```python
from build123d import *

# Parameters (mm, degrees)
SKETCH1_W                      = 260
SKETCH1_H                      = 49
BOSS_EXTRUDE1_DEPTH            = 6
SKETCH2_W                      = 117
SKETCH2_H                      = 6
CUT_EXTRUDE1_DEPTH             = 140.057542046
SKETCH5_W                      = 3.4
SKETCH5_H                      = 6
CUT_EXTRUDE2_REACH             = 141.058
SKETCH6_W                      = 6
SKETCH6_H                      = 23
SKETCH7_W                      = 80
SKETCH7_H                      = 6
BOSS_EXTRUDE2_DEPTH            = 6
SKETCH8_R                      = 20
SKETCH8_R_2                    = 8.5
CUT_EXTRUDE3_DEPTH             = 6
SKETCH9_R                      = 5.75
BOSS_EXTRUDE3_DEPTH            = 6
CIRPATTERN1_COUNT              = 5
SKETCH11_W                     = 1.4351
SKETCH11_H                     = 6
F_6_40_TAPPED_HOLE1_AT_2_COUNT = 2
F_6_40_TAPPED_HOLE1_AT_2_PITCH = 32
F_6_40_TAPPED_HOLE1_AT_3_COUNT = 2
F_6_40_TAPPED_HOLE1_AT_3_PITCH = 45.254833996
F_6_40_TAPPED_HOLE1_AT_4_COUNT = 2
F_6_40_TAPPED_HOLE1_AT_4_PITCH = 32
SKETCH12_R                     = 1.4351
SKETCH12_R_2                   = 3.4
SKETCH12_R_3                   = 5.75
CUT_EXTRUDE4_DEPTH             = 6


with BuildPart() as part:
    # Sketch1 → Boss-Extrude1 (new body)
    with BuildSketch(Plane.XY):
        with Locations((0, 24.5)):
            Rectangle(SKETCH1_W, SKETCH1_H)
    extrude(amount=BOSS_EXTRUDE1_DEPTH)

    # Sketch2 → Cut-Extrude1 (cut, through all)
    with BuildSketch(Plane(origin=(0, 0, 0), x_dir=(-1, 0, 0), z_dir=(0, 0, -1))):
        with Locations((-71.5, 46)):
            Rectangle(SKETCH2_W, SKETCH2_H)
        with Locations((71.5, 46)):
            Rectangle(SKETCH2_W, SKETCH2_H)
    extrude(amount=-CUT_EXTRUDE1_DEPTH, mode=Mode.SUBTRACT)

    # Sketch5 → M8x1.25 Tapped Hole1 (revolve, cut)
    with BuildSketch(Plane(origin=(0, 39, 0), x_dir=(0, 1, 0), z_dir=(1, 0, 0))):
        with Locations((1.7, 3)):
            Rectangle(SKETCH5_W, SKETCH5_H)
    revolve(axis=Axis((0, 39, -6.35), (0, 0, 1)), mode=Mode.SUBTRACT)

    # Sketch6 → Cut-Extrude2 (cut, up to next)
    with BuildSketch(Plane(origin=(0, 0, 0), x_dir=(-1, 0, 0), z_dir=(0, 0, -1)), mode=Mode.PRIVATE) as cut_extrude2_sk1:
        with Locations((-127, 31.5)):
            Rectangle(SKETCH6_W, SKETCH6_H)
    cut_extrude2_tool1 = extrude(cut_extrude2_sk1.sketch, amount=-CUT_EXTRUDE2_REACH, mode=Mode.PRIVATE) & part.part
    # Sketch6 → Cut-Extrude2 (cut, up to next)
    with BuildSketch(Plane(origin=(0, 0, 0), x_dir=(-1, 0, 0), z_dir=(0, 0, -1)), mode=Mode.PRIVATE) as cut_extrude2_sk2:
        with Locations((127, 31.5)):
            Rectangle(SKETCH6_W, SKETCH6_H)
    cut_extrude2_tool2 = extrude(cut_extrude2_sk2.sketch, amount=-CUT_EXTRUDE2_REACH, mode=Mode.PRIVATE) & part.part
    add(cut_extrude2_tool1.solids().sort_by_distance((127, 31.5, 0))[0], mode=Mode.SUBTRACT)
    add(cut_extrude2_tool2.solids().sort_by_distance((-127, 31.5, 0))[0], mode=Mode.SUBTRACT)

    # Sketch7 → Boss-Extrude2 (add)
    with BuildSketch(Plane(origin=(0, 0, 0), x_dir=(-1, 0, 0), z_dir=(0, 0, -1))):
        with Locations((0, -3)):
            Rectangle(SKETCH7_W, SKETCH7_H)
    extrude(amount=-BOSS_EXTRUDE2_DEPTH)

    # Sketch8 → Cut-Extrude3 (cut)
    with BuildSketch(Plane(origin=(0, 0, 0), x_dir=(-1, 0, 0), z_dir=(0, 0, -1))):
        with Locations((-85, 21.5)):
            Circle(SKETCH8_R)
        with Locations((-85, 21.5)):
            Circle(SKETCH8_R_2, mode=Mode.SUBTRACT)
    extrude(amount=-CUT_EXTRUDE3_DEPTH, mode=Mode.SUBTRACT)


with BuildPart() as cut_extrude3_piece_1:
    # of the separate pieces the step leaves, piece 1, a body of its own (cut_extrude3_pieces)
    add(part.part.solids().sort_by_distance((130, 0, 0))[0])



with BuildPart() as cut_extrude3_piece_2:
    # of the separate pieces the step leaves, piece 2, a body of its own (cut_extrude3_pieces)
    add(part.part.solids().sort_by_distance((76.5, 21.5, 0))[0])


with BuildPart() as cut_extrude3_piece_1_1:
    add(cut_extrude3_piece_1.part)

    add(cut_extrude3_piece_2.part)  # Boss-Extrude3 merges Cut-Extrude3 piece 2
    # Sketch9 → Boss-Extrude3 (add)
    with BuildSketch(Plane(origin=(0, 0, 0), x_dir=(-1, 0, 0), z_dir=(0, 0, -1))):
        with BuildLine():
            ThreePointArc((-100.761482737, 35.377163324), (-88.82060414, 26.758610463), (-93.327400585, 40.778340164))
            ThreePointArc((-93.327400585, 40.778340164), (-97.343490298, 38.489356882), (-100.761482737, 35.377163324))
        make_face()
        with Locations((-93.375939845, 33.02849217)):
            Circle(SKETCH9_R, mode=Mode.SUBTRACT)
    boss_extrude3 = extrude(amount=-BOSS_EXTRUDE3_DEPTH)

    # CirPattern1: Boss-Extrude3 ×5 about axis
    cirpattern1_axis = Axis((85, 21.5, 0), (0, 0, -1))
    for i in range(1, CIRPATTERN1_COUNT):
        add(boss_extrude3.rotate(cirpattern1_axis, i * 360 / CIRPATTERN1_COUNT))

    # Sketch11 → #6-40 Tapped Hole1 (revolve, cut)
    with BuildSketch(Plane(origin=(101, 37.5, 0), x_dir=(0, 1, 0), z_dir=(1, 0, 0))):
        with Locations((0.71755, 3)):
            Rectangle(SKETCH11_W, SKETCH11_H)
    f_6_40_tapped_hole1 = revolve(axis=Axis((101, 37.5, -6.35), (0, 0, 1)), mode=Mode.SUBTRACT)

    # #6-40 Tapped Hole1 at 2: #6-40 Tapped Hole1 ×2
    with Locations(*[(-i * F_6_40_TAPPED_HOLE1_AT_2_PITCH, 0, 0) for i in range(1, F_6_40_TAPPED_HOLE1_AT_2_COUNT)]):
        add(f_6_40_tapped_hole1, mode=Mode.SUBTRACT)

    # #6-40 Tapped Hole1 at 3: #6-40 Tapped Hole1 ×2
    with Locations(*[Vector(-0.7071067811865476, -0.7071067811865476, 0) * (i * F_6_40_TAPPED_HOLE1_AT_3_PITCH) for i in range(1, F_6_40_TAPPED_HOLE1_AT_3_COUNT)]):
        add(f_6_40_tapped_hole1, mode=Mode.SUBTRACT)

    # #6-40 Tapped Hole1 at 4: #6-40 Tapped Hole1 ×2
    with Locations(*[(0, -i * F_6_40_TAPPED_HOLE1_AT_4_PITCH, 0) for i in range(1, F_6_40_TAPPED_HOLE1_AT_4_COUNT)]):
        add(f_6_40_tapped_hole1, mode=Mode.SUBTRACT)

    # Sketch12 → Cut-Extrude4 (cut)
    with BuildSketch(Plane(origin=(0, 0, 0), x_dir=(-1, 0, 0), z_dir=(0, 0, -1))):
        with Locations(Location((101, 37.5, 0), (0, 0, 180))):
            Circle(SKETCH12_R)
        with Locations((0, 39)):
            Circle(SKETCH12_R_2)
        with Locations((-93.375939845, 33.02849217)):
            Circle(SKETCH12_R_3)
        with Locations(Location((-76.624060155, 33.02849217, 0), (0, 0, 288))):
            Circle(SKETCH12_R_3)
        with Locations(Location((-71.447444643, 17.09650783, 0), (0, 0, 216))):
            Circle(SKETCH12_R_3)
        with Locations(Location((-85, 7.25, 0), (0, 0, 144))):
            Circle(SKETCH12_R_3)
        with Locations(Location((-98.552555357, 17.09650783, 0), (0, 0, 72))):
            Circle(SKETCH12_R_3)
        with Locations((-101, 5.5)):
            Circle(SKETCH12_R)
        with Locations((-69, 5.5)):
            Circle(SKETCH12_R)
        with Locations((-69, 37.5)):
            Circle(SKETCH12_R)
        with Locations((-101, 37.5)):
            Circle(SKETCH12_R)
        with Locations(Location((69, 37.5, 0), (0, 0, 180))):
            Circle(SKETCH12_R)
        with Locations(Location((69, 5.5, 0), (0, 0, 180))):
            Circle(SKETCH12_R)
        with Locations(Location((101, 5.5, 0), (0, 0, 180))):
            Circle(SKETCH12_R)
        with Locations(Location((98.552555357, 17.09650783, 0), (0, 0, 180))):
            Circle(SKETCH12_R_3)
        with Locations(Location((85, 7.25, 0), (0, 0, 180))):
            Circle(SKETCH12_R_3)
        with Locations(Location((71.447444643, 17.09650783, 0), (0, 0, 180))):
            Circle(SKETCH12_R_3)
        with Locations(Location((76.624060155, 33.02849217, 0), (0, 0, 180))):
            Circle(SKETCH12_R_3)
        with Locations(Location((93.375939845, 33.02849217, 0), (0, 0, 180))):
            Circle(SKETCH12_R_3)
        with BuildLine():
            ThreePointArc((-78.722018184, 40.489127003), (-83.633443041, 36.334706252), (-83.715608088, 29.902400694))
            ThreePointArc((-83.715608088, 29.902400694), (-85, 30), (-86.284391912, 29.902400694))
            ThreePointArc((-86.284391912, 29.902400694), (-86.366556959, 36.334706252), (-91.277981816, 40.489127003))
            ThreePointArc((-91.277981816, 40.489127003), (-85, 41.5), (-78.722018184, 40.489127003))
        make_face()
        with BuildLine():
            ThreePointArc((-65.000263954, 21.397247437), (-65.978869674, 27.680339887), (-68.880270097, 33.338678467))
            ThreePointArc((-68.880270097, 33.338678467), (-71.313645276, 27.383849239), (-77.405740996, 25.318013906))
            ThreePointArc((-77.405740996, 25.318013906), (-76.916019611, 24.126644452), (-76.611943139, 22.87495531))
            ThreePointArc((-76.611943139, 22.87495531), (-70.469066627, 24.784503438), (-65.000263954, 21.397247437))
        make_face()
        with BuildLine():
            ThreePointArc((-78.917465173, 2.447368421), (-73.244294954, 5.319660113), (-68.759477215, 9.827578672))
            ThreePointArc((-68.759477215, 9.827578672), (-75.174810639, 10.301712562), (-79.022097904, 15.45726167))
            ThreePointArc((-79.022097904, 15.45726167), (-80.003825356, 14.623355548), (-81.100287673, 13.947368421))
            ThreePointArc((-81.100287673, 13.947368421), (-77.385946247, 8.695228508), (-78.917465173, 2.447368421))
        make_face()
        with BuildLine():
            ThreePointArc((-93.388056861, 22.87495531), (-99.530933373, 24.784503438), (-104.999736046, 21.397247437))
            ThreePointArc((-104.999736046, 21.397247437), (-104.021130326, 27.680339887), (-101.119729903, 33.338678467))
            ThreePointArc((-101.119729903, 33.338678467), (-98.686354724, 27.383849239), (-92.594259004, 25.318013906))
            ThreePointArc((-92.594259004, 25.318013906), (-93.083980389, 24.126644452), (-93.388056861, 22.87495531))
        make_face()
        with BuildLine():
            ThreePointArc((-101.240522785, 9.827578672), (-96.755705046, 5.319660113), (-91.082534827, 2.447368421))
            ThreePointArc((-91.082534827, 2.447368421), (-92.614053753, 8.695228508), (-88.899712327, 13.947368421))
            ThreePointArc((-88.899712327, 13.947368421), (-89.996174644, 14.623355548), (-90.977902096, 15.45726167))
            ThreePointArc((-90.977902096, 15.45726167), (-94.825189361, 10.301712562), (-101.240522785, 9.827578672))
        make_face()
        with BuildLine():
            ThreePointArc((88.899712327, 13.947368421), (92.614053753, 8.695228508), (91.082534827, 2.447368421))
            ThreePointArc((91.082534827, 2.447368421), (96.755705046, 5.319660113), (101.240522785, 9.827578672))
            ThreePointArc((101.240522785, 9.827578672), (94.825189361, 10.301712562), (90.977902096, 15.45726167))
            ThreePointArc((90.977902096, 15.45726167), (89.996174644, 14.623355548), (88.899712327, 13.947368421))
        make_face()
        with BuildLine():
            ThreePointArc((92.594259004, 25.318013906), (93.083980389, 24.126644452), (93.388056861, 22.87495531))
            ThreePointArc((93.388056861, 22.87495531), (99.530933373, 24.784503438), (104.999736046, 21.397247437))
            ThreePointArc((104.999736046, 21.397247437), (104.021130326, 27.680339887), (101.119729903, 33.338678467))
            ThreePointArc((101.119729903, 33.338678467), (98.686354724, 27.383849239), (92.594259004, 25.318013906))
        make_face()
        with BuildLine():
            ThreePointArc((79.022097904, 15.45726167), (75.174810639, 10.301712562), (68.759477215, 9.827578672))
            ThreePointArc((68.759477215, 9.827578672), (73.244294954, 5.319660113), (78.917465173, 2.447368421))
            ThreePointArc((78.917465173, 2.447368421), (77.385946247, 8.695228508), (81.100287673, 13.947368421))
            ThreePointArc((81.100287673, 13.947368421), (80.003825356, 14.623355548), (79.022097904, 15.45726167))
        make_face()
        with BuildLine():
            ThreePointArc((77.405740996, 25.318013906), (71.313645276, 27.383849239), (68.880270097, 33.338678467))
            ThreePointArc((68.880270097, 33.338678467), (65.978869674, 27.680339887), (65.000263954, 21.397247437))
            ThreePointArc((65.000263954, 21.397247437), (70.469066627, 24.784503438), (76.611943139, 22.87495531))
            ThreePointArc((76.611943139, 22.87495531), (76.916019611, 24.126644452), (77.405740996, 25.318013906))
        make_face()
        with BuildLine():
            ThreePointArc((78.722018184, 40.489127003), (85, 41.5), (91.277981816, 40.489127003))
            ThreePointArc((91.277981816, 40.489127003), (86.366556959, 36.334706252), (86.284391912, 29.902400694))
            ThreePointArc((86.284391912, 29.902400694), (85, 30), (83.715608088, 29.902400694))
            ThreePointArc((83.715608088, 29.902400694), (83.633443041, 36.334706252), (78.722018184, 40.489127003))
        make_face()
    extrude(amount=-CUT_EXTRUDE4_DEPTH, mode=Mode.SUBTRACT)


solid = cut_extrude3_piece_1_1.part
```
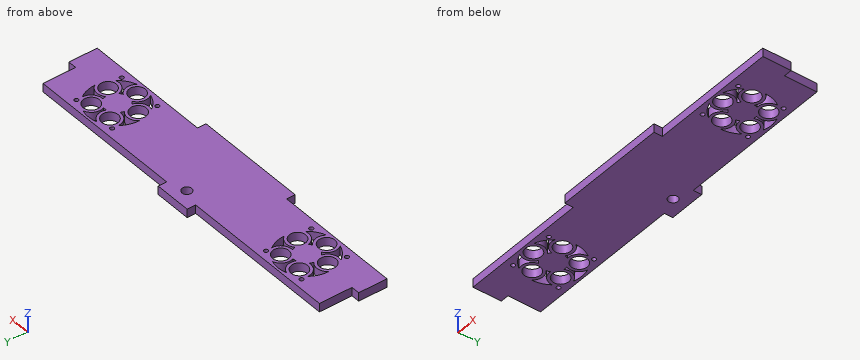
Source: CAD feature listing. Evaluate the final solid. Frame: model axes, mm. Give positions to 0.01 mm unless a question says otherwise; leave off trailing zeros. Loops run counter-clockwise (first coordinate to the right, second up) from the corner with the lowest first, then second, coordinate; pieces in that order, holes last. Notation, with made-up numbers: (79.5, 65.5) -> (112.5, 65.5) arc R7 cw to (112.5, 72.5) -> close; hole circle Ø3 at (84, 4.25). An arc over 180 degrees is marked (long way). Use a Markdown table: item, result. Add a question column.
(1) Section query B-B (x = 33.5). Output: boundary loops of the cut face in (y, z), then the cut area to 3 significant figures.
(2) Section query C-C (z = 3.4). Count the separate pieces of the cut face and the enclosed holes in it, then the cut area to 3 significant figures.
(3) First-contact query: pin 1 Ø1.7 at (x, y) = (69, 37.5) entering from +Z; pin 2 Ø1.5 at (x, z) = (-53.5, 0.5) entering from -Y; pin 3 Ø3 at (x, z) = (-126.5, 2.5) entering from +Y. Flat tips, straight axial feed; report the tip coordinate or a pass-through.
(4) Ray query, line 1 (Y direction, x = 92, z = 2.35) (3 decimals); line 2 (Y direction, x = 91.5, z = 3.1); line 3 (X direction, y = 46, z = 5). Return the intervals inside material, ascending.
(5) Section query A-A (x = 0). Output: boundary loops of the cut face in (y, z).
Checked values:
| question | item | result |
|---|---|---|
| 1 | outline | (-6, 0) -> (43, 0) -> (43, 6) -> (-6, 6) -> close |
| 1 | area | 294 mm^2 |
| 2 | separate pieces | 1 |
| 2 | enclosed holes | 29 |
| 2 | area | 9,960 mm^2 |
| 3 | pin 1 | through |
| 3 | pin 2 | y = 0 |
| 3 | pin 3 | y = 20 |
| 4 | line 1 | 0 to 2.765, 3.924 to 10.576, 12.958 to 27.446, 38.611 to 43 |
| 4 | line 2 | 0 to 2.59, 3.03 to 11.47, 13.88 to 27.59, 38.46 to 43 |
| 4 | line 3 | -13 to 13 |
| 5 | outline | (-6, 0) -> (35.6, 0) -> (35.6, 6) -> (-6, 6) -> close; (42.4, 0) -> (49, 0) -> (49, 6) -> (42.4, 6) -> close |
